from build123d import *

# Parameters (mm, degrees)
SKETCH_1_R      = 25
SKETCH_1_R_2    = 2
SKETCH_1_R_3    = 5
EXTRUDE_1_DEPTH = 3
SKETCH_2_W      = 5
SKETCH_2_H      = 12
EXTRUDE_2_DEPTH = 3
FILLET_1_R      = 1


with BuildPart() as part:
    # 草图1 → 凸台-拉伸1 (new body)
    with BuildSketch(Plane(origin=(0, 0, 0), x_dir=(1, 0, 0), z_dir=(0, 1, 0))):
        with Locations(Location((0, 0, 0), (0, 0, 270))):
            Circle(SKETCH_1_R)
        with Locations(Location((0, 19, 0), (0, 0, 270))):
            Circle(SKETCH_1_R_2, mode=Mode.SUBTRACT)
        with Locations(Location((16.454482672, 9.5, 0), (0, 0, 270))):
            Circle(SKETCH_1_R_2, mode=Mode.SUBTRACT)
        with Locations(Location((16.454482672, -9.5, 0), (0, 0, 270))):
            Circle(SKETCH_1_R_2, mode=Mode.SUBTRACT)
        with Locations(Location((0, -19, 0), (0, 0, 270))):
            Circle(SKETCH_1_R_2, mode=Mode.SUBTRACT)
        with Locations(Location((-16.454482672, -9.5, 0), (0, 0, 270))):
            Circle(SKETCH_1_R_2, mode=Mode.SUBTRACT)
        with Locations(Location((-16.454482672, 9.5, 0), (0, 0, 270))):
            Circle(SKETCH_1_R_2, mode=Mode.SUBTRACT)
        with Locations(Location((0, 0, 0), (0, 0, 270))):
            Circle(SKETCH_1_R_3, mode=Mode.SUBTRACT)
    extrude(amount=EXTRUDE_1_DEPTH)

    # 草图2 → 凸台-拉伸2 (add)
    with BuildSketch(Plane(origin=(0, 3, 0), x_dir=(1, 0, 0), z_dir=(0, 1, 0))):
        Rectangle(SKETCH_2_W, SKETCH_2_H)
    extrude(amount=-EXTRUDE_2_DEPTH)

    # 圆角1
    fillet_1_edges = [part.edges().sort_by_distance(p)[0] for p in [
        (-2.5, 1.5, 4.330127019),
        (-2.5, 1.5, -4.330127019),
        (2.5, 1.5, -4.330127019),
        (2.5, 1.5, 4.330127019),
    ]]
    fillet(fillet_1_edges, radius=FILLET_1_R)


solid = part.part
Can you work these out from the model? Positions are in its coordinate system, mm. A direction names the side the tool comes from. Round coordinates to 2 decimals unless told otherwise and drop trailing zeros. Loops run counter-clockwise (first coordinate to the right, second up) from the corner with the lowest first, then second, coordinate; pieces in that order, holes last. Notation, with made-up numbers: (3, 70) - (15, 70) arc R28 ccw to (15, 92) - close; hole circle Ø8 at (82, 4). An arc over 180 degrees is marked (long way). Answer in a Markdown table with one row per item. Add a question column.
Q1. I want a section at C-C on y = 0.55. Count the separate pieces of the cut face and the enclosed holes in it, and give its area (3 significant figures).
Q2. I want a section at D-D on z = -19. List the corners of the cut face in (x, y) for me, and give its area (3 significant figures).
Q3. Which directions (+Z, -Z, +X, -X, +Y, -Y) give clear straight access to the entire face, cutting with the end or side of a thin tool? Please do faces 1 (the flat face through (0, 0, 0)), 2 (the cylindrical face through (-3.23, 1.48, -2.9)).
Q4. We'd pull the mould along X, two halves only. Please class faces 3 (the flat face through (0, 3, 0)), 4 (the cylindrical face through (-3.23, 1.48, 2.9)), 5 (the cylindrical face through (7.509, 1.479, 23.846)): pulls with the +X half, pulls with the -X half, needs draft (parallel to the pull), parting line crosses it, or undercut.
Q5. I want a section at A-A on x = 0. List the corners of the cut face in (y, z) for me.
Q6. I need wall thicknesses on L1, parallel to X at y = 1.25, z = 9.5; L2, parallel to Z at x = 18, y = 2.6; L3, parallel to X at y = 2.5, z = -9. Which ranges of each line are inside material? Lowest first, please.
Q7. For pin 1 Ø5 at (x, z) = (-16.45, 9.5) entering from -Y, with a flat end and sliding along its axis, tell me the tip position at first contact or that it passes through.
Q8. I want a section at B-B on z = 0. List the corners of the cut face in (x, y) for me, and give its area (3 significant figures).
A:
| question | item | result |
|---|---|---|
| 1 | separate pieces | 1 |
| 1 | enclosed holes | 8 |
| 1 | area | 1,860 mm^2 |
| 2 | outline | (-16.25, 0) - (-2, 0) - (-2, 3) - (-16.25, 3) - close; (2, 0) - (16.25, 0) - (16.25, 3) - (2, 3) - close |
| 2 | area | 85.5 mm^2 |
| 3 | face 1 | +Z, -Z, +X, -X, -Y |
| 3 | face 2 | +Y, -Y |
| 4 | face 3 | needs draft |
| 4 | face 4 | undercut |
| 4 | face 5 | parting line crosses it |
| 5 | outline | (0, -25) - (3, -25) - (3, -21) - (0, -21) - close; (0, -17) - (3, -17) - (3, 17) - (0, 17) - close; (0, 21) - (3, 21) - (3, 25) - (0, 25) - close |
| 6 | L1 | -23.12 to -18.45, -14.45 to 14.45, 18.45 to 23.12 |
| 6 | L2 | -17.35 to -10.77, -8.23 to 8.23, 10.77 to 17.35 |
| 6 | L3 | -23.32 to -18.39, -14.52 to 14.52, 18.39 to 23.32 |
| 7 | pin 1 | y = 0 |
| 8 | outline | (-25, 0) - (-5, 0) - (-5, 3) - (-25, 3) - close; (-2.5, 0) - (2.5, 0) - (2.5, 3) - (-2.5, 3) - close; (5, 0) - (25, 0) - (25, 3) - (5, 3) - close |
| 8 | area | 135 mm^2 |
